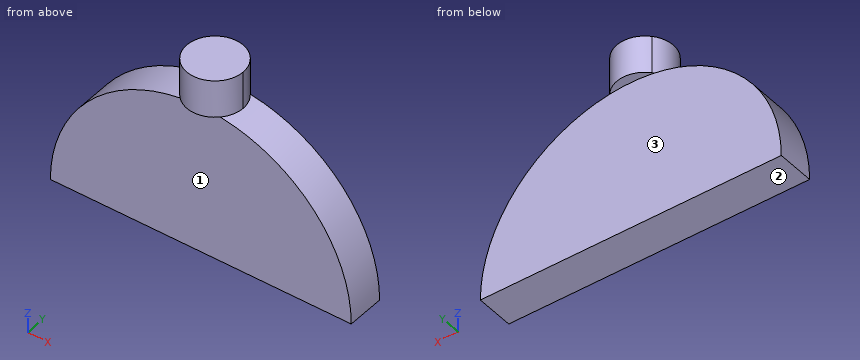
```python
from build123d import *

# Parameters (mm, degrees)
F1_DEPTH = 50.8
F4_DEPTH = 50.8


with BuildPart() as f1:
    # F0 (on Front) → F1 (new body)
    with BuildSketch(Plane.XZ):
        with BuildLine():
            ThreePointArc((406.4, 0), (203.2, 203.2), (0, 0))
            Line((0, 0), (406.4, 0))
        make_face()
    extrude(amount=F1_DEPTH)

    # F3 (on offset) → F4 (join)
    with BuildSketch(Plane.XY.offset(202.946)):
        with BuildLine():
            ThreePointArc((174.801937, 0), (189.605078, -60.991967), (241.3, -25.4))
            ThreePointArc((241.3, -25.4), (216.794922, 10.191967), (174.801937, 0))
        make_face()
    extrude(amount=F4_DEPTH)


solid = f1.part
```
Input: part model. Units: mm. Frame: model coordinates. Face numbers are marked on the shaded views. A direction names the side the tool comes from. Give positions to 0.01 mm unless a question says otherwise; leave off trailing zeros. Order: outer loops, then holes, each group sorted by start corner. A loop starts at its lowest first (then second) coordinate and runs counter-clockwise, first axis right, second up.
1. Section A-A on x = 203.2. Return the cut outline in (y, z), and give its area (3 significant figures).
Derived:
outline: (-63.5, 202.95) - (-50.8, 202.95) - (-50.8, 0) - (0, 0) - (0, 202.95) - (12.7, 202.95) - (12.7, 253.75) - (-63.5, 253.75) - close
area: 14,200 mm2
2. Pin query (flat end, axial travel): pin 1 (3 mm diameter, centred on x = 328.5, z = 94.5, fed in from +Y); pin 2 (10 mm diameter, centred on x = 115.5, y = -0.5, fed in from +Z); pin 3 (1.5 mm diameter, centred on y = -1.5, z = 167.5, fed in from -X). Return the tip coordinate at first contact, or that it passes through.
Derived:
pin 1: stops at y = 0
pin 2: stops at z = 185.61
pin 3: stops at x = 87.08
3. Material intervals for L1, parallel to Y at x = 101, z = 63; L2, parallel to Z at x = 234, y = -13.5; L3, parallel to Z at x = 218, y = -39.5, sorted ascending.
Derived:
L1: y = -50.8 to 0
L2: z = 0 to 200.85, 202.95 to 253.75
L3: z = 0 to 202.66, 202.95 to 253.75
4. Section C-C on z = 235.5. Return the cut outline in (x, y).
Derived:
outline: circle Ø76.2 at (203.2, -25.4)
5. Reachability of the marked faces 1, 2 and 3 from +Z, -Z, +X, -X, +Y, -Y: full face, straight path, thin tool, end or side. Return the list, or none.
Derived:
face 1: -Z, +X, -X, -Y
face 2: -Z, +X, -X, +Y, -Y
face 3: -Z, +X, -X, +Y
6. Section B-B on y = -43. Return the cut outline in (x, z).
Derived:
outline: (0, 0) - (406.4, 0) arc R203.2 ccw to (213.36, 202.95) - (236.99, 202.95) - (236.99, 253.75) - (169.41, 253.75) - (169.41, 202.95) - (193.04, 202.95) arc R203.2 ccw to start
7. Section D-D on z = 182.5. Return the cut outline in (x, y), and give its area (3 significant figures).
Derived:
outline: (113.85, -50.8) - (292.55, -50.8) - (292.55, 0) - (113.85, 0) - close
area: 9,080 mm2
